For this review, take the finished solid that the model builds, in its own axes (mm). A direction names the side the tool comes from. Coordinates: 2 decimals unless noted, no trailing zeros. Loops run counter-clockwise (first coordinate to the right, second up) from the corner with the lowest first, then second, coordinate; pieces in that order, holes last.
1. Take a section at D-D, the plane z = 27. State the section outline as (x, y) points.
2. Take a section at B-B, the plane x = 45.5. State the section outline as (y, z) points.
3. Clearance check with flat-ended pins moving along their axes: P1, Ø5, axis at y = 21.5, z = 13, coming from the +X side; P2, Ø3, axis at x = 43.5, z = 5, coming from the +Y side; P3, Ø10, axis at y = -5, z = 8.5, coming from the +X side. State where each tip first meets the part, or that it passes through.
4. Take a section at C-C, the plane y = -12. State the section outline as (x, z) points, then the cut area to 3 significant figures.
5. Mouldability with a two-part tool opening along Z and no side actions: class faces 5 (the face through (-2, 16.237, 15)), 6 (the face through (-11, 27, 15)), 7 (the face through (-2.465, 18.652, 10.856)), 8 (the face through (30.819, 11.028, 5.944)) as pulls with the +Z half, pulls with the -Z half, needs draft (parallel to the pull), parting line crosses it, or undercut.
6. To check wall thickness, follow probe 1 along Y at (x, z) = (-10.25, 15); probe 2 along Z at (x, y) = (-8, 21); probe 3 along Y at (x, z) = (-15, 15). State the ranges of each line that lie inside material, in increasing order.
7. Take a section at A-A, the plane z = 15. Count the separate pieces of the cut face and the enclosed holes in it, then the cut area to 3 significant figures.
8. Machinability: for faces 1 (the face through (2, 0, 10)), 2 (the face through (32.143, -8.392, 5.714)), 3 (the face through (28, 15, 6)), 4 (the face through (-5, -17.8, 16.1)), which of the approach directions +Z, -Z, +X, -X, +Y, -Y give a long, thin tool a straight path to every point of the face, cutting with its end or side? Answer none if there is none.
```python
from build123d import *

# Parameters (mm, degrees)
PRISM_DEPTH                         = 5
CYLINDER_R                          = 3.2
CYLINDER_DEPTH                      = 30
FUSION_PLACEMENT_ANGLE              = 90
EXTRUDE002_DEPTH                    = 30
BOX_W                               = 80
BOX_H                               = 40
BOX_DEPTH                           = 10
SKETCH_AS_DRAWN_R                   = 0.9
EXTRUDE_DEPTH                       = 15
EXTRUDE_ONTO_SKETCH_PLACEMENT_ANGLE = 15.945396
EXTRUDE004_DEPTH                    = 30
EXTRUDE003_DEPTH                    = 30


with BuildPart() as prisma:
    # Prism → Prism (new body)
    with BuildSketch(Plane.XY):
        Polygon((5.5, 0), (2.75, 4.76314), (-2.75, 4.76314), (-5.5, 0), (-2.75, -4.76314), (2.75, -4.76314), align=None)
    extrude(amount=PRISM_DEPTH)


with BuildPart() as obj1:
    # Cylinder → Cylinder (new body)
    with BuildSketch(Plane.XY):
        Circle(CYLINDER_R)
    extrude(amount=CYLINDER_DEPTH)

    # Fusion: union Prisma
    add(prisma.part)


with BuildPart() as obj1_1:
    # Fusion placement: moved
    add(obj1.part.moved(Location((0, -21, 15))).rotate(Axis((0, -21, 15), (0, -1, 0)), FUSION_PLACEMENT_ANGLE))


with BuildPart() as obj2:
    # Clone base: copy of obj1
    add(obj1_1.part)


with BuildPart() as obj2_1:
    # Clone placement: moved
    add(obj2.part.moved(Location((0, 42, 0))))


with BuildPart() as obj3:
    # Fusion001 base: copy of obj1
    add(obj1_1.part)

    # Fusion001: union obj2
    add(obj2_1.part)


with BuildPart() as obj4:
    # Sketch002 → Extrude002 (new body)
    with BuildSketch(Plane.XY):
        with BuildLine():
            Line((-20, 27), (-1, 27))
            ThreePointArc((0, 26), (-0.292893, 26.707107), (-1, 27))
            Line((0, 26), (0, -26))
            ThreePointArc((-1, -27), (-0.292893, -26.707107), (0, -26))
            Line((-1, -27), (-20, -27))
            Line((-20, -27), (-20, -15))
            ThreePointArc((-20, -15), (-11.949874, 0), (-20, 15))
            Line((-20, 15), (-20, 27))
        make_face()
    extrude(amount=EXTRUDE002_DEPTH)


with BuildPart() as obj5:
    # Box → Box (new body)
    with BuildSketch(Plane(origin=(0, -35, -10), x_dir=(1, 0, 0), z_dir=(0, 0, 1))):
        with Locations((40, 20)):
            Rectangle(BOX_W, BOX_H)
    extrude(amount=BOX_DEPTH)


with BuildPart() as obj6:
    # Sketch as drawn → Extrude (new)
    with BuildSketch(Plane.XY):
        with BuildLine():
            Line((32, -28), (28, -28))
            Line((28, -28), (28, -24))
            ThreePointArc((32, -24), (30, -22), (28, -24))
            Line((32, -28), (32, -24))
        make_face()
        with Locations((30, -24)):
            Circle(SKETCH_AS_DRAWN_R, mode=Mode.SUBTRACT)
    extrude(amount=-EXTRUDE_DEPTH)


with BuildPart() as obj6_1:
    # Extrude onto Sketch placement: moved
    add(obj6.part.moved(Location((5.54717, 0, 19.415094))).rotate(Axis((5.54717, 0, 19.415094), (0, 1, 0)), EXTRUDE_ONTO_SKETCH_PLACEMENT_ANGLE))


with BuildPart() as cut:
    # Part__Mirroring: instance of obj6
    add(obj6_1.part.mirror(Plane(origin=(0, 0, 0), x_dir=(1, 0, 0), z_dir=(0, 1, 0))))


with BuildPart() as cut_1:
    # Part__Mirroring placement: moved
    add(cut.part.moved(Location((0, -30, 0))))

    # Fusion002: union obj6
    add(obj6_1.part)

    # Cut: cut obj5
    add(obj5.part, mode=Mode.SUBTRACT)


with BuildPart() as obj7:
    # Sketch004 → Extrude004 (new body)
    with BuildSketch(Plane(origin=(0, 0, 0), x_dir=(1, 0, 0), z_dir=(0, 0, -1))):
        with BuildLine():
            Line((4, 28), (66, 28))
            ThreePointArc((68, 26), (67.414214, 27.414214), (66, 28))
            Line((68, 26), (68, 4))
            ThreePointArc((66, 2), (67.414214, 2.585786), (68, 4))
            Line((66, 2), (4, 2))
            ThreePointArc((2, 4), (2.585786, 2.585786), (4, 2))
            Line((2, 4), (2, 26))
            ThreePointArc((4, 28), (2.585786, 27.414214), (2, 26))
        make_face()
    extrude(amount=EXTRUDE004_DEPTH)


with BuildPart() as obj7_1:
    # Extrude004 placement: moved
    add(obj7.part.moved(Location((0, 0, 30))))


with BuildPart() as solar_halter:
    # Sketch003 → Extrude003 (new body)
    with BuildSketch(Plane.XZ):
        Polygon((0, 0), (0, 21), (70, 1), (70, 0), align=None)
    extrude(amount=EXTRUDE003_DEPTH)

    # Cut001: cut obj7
    add(obj7_1.part, mode=Mode.SUBTRACT)

    # Fusion003: union Cut
    add(cut_1.part)


with BuildPart() as solar_halter_1:
    # Fusion003 placement: moved
    add(solar_halter.part.moved(Location((0, 15, 0))))

    # Fusion004: union obj4
    add(obj4.part)

    # Cut002: cut obj3
    add(obj3.part, mode=Mode.SUBTRACT)


solid = solar_halter_1.part
```
Results list:
1. outline: (-20, -27) - (-1, -27) arc R1 ccw to (0, -26) - (0, 26) arc R1 ccw to (-1, 27) - (-20, 27) - (-20, 15) arc R18 cw to (-20, -15) - close
2. outline: (-15, 0) - (-13, 0) - (-13, 8) - (-15, 8) - close; (13, 0) - (15, 0) - (15, 8) - (13, 8) - close
3. P1: stops at x = -5
3. P2: stops at y = 15
3. P3: stops at x = 36.32
4. outline: (-16.53, 0) - (2.27, 0) - (2.27, 20.35) - (0, 21) - (0, 30) - (-16.53, 30) - close; (29.12, 0) - (33.28, 0) - (36.32, 10.62) - (32.47, 11.72) - close; (67.73, 0) - (70, 0) - (70, 1) - (67.73, 1.65) - close
4. area: 592 mm2
5. face 5: undercut
5. face 6: needs draft
5. face 7: undercut
5. face 8: pulls with the +Z half
6. probe 1: y = -27 to -24.2, -17.8 to 17.8, 24.2 to 27
6. probe 2: z = 0 to 11.8, 18.2 to 30
6. probe 3: y = -27 to -24.2, -17.8 to -10.03, 10.03 to 17.8, 24.2 to 27
7. separate pieces: 3
7. enclosed holes: 0
7. area: 760 mm2
8. face 1: +Z, -Z
8. face 2: none
8. face 3: +Z, -Z, +X, +Y
8. face 4: +X
